CAD build for the part. Positions are in the model's coordinates, mm. A direction names the side the tool comes from. Round coordinates to 2 decimals unless told otherwise and drop trailing zeros. Write each loop counter-clockwise with the first axis right and the second up, starting at its lowest first coordinate (ties: lowest second). Pieces come first, ordered by that corner, then holes. Notation, with made-up numbers: (42, -35) - (84, -35) arc R12 ccw to (84, -27) - close; hole circle Ø1 at (80, 78.5). An arc over 180 degrees is marked (long way). Answer in a Markdown table with one row per item.
```python
from build123d import *

# Parameters (mm, degrees)
F0_R        = 10.025
F0_R_2      = 4.5
F1_DEPTH    = 1.5
F0_R_3      = 11.025
F1_FACE_R   = 10.025
F1_FACE_R_2 = 4.5
F2_DEPTH    = 2
F3_DEPTH    = 2
F4_DEPTH    = 1.5
F5_DEPTH    = 1.5
F6_DEPTH    = 2
F7_DEPTH    = 1.5


with BuildPart() as f1:
    # F0 (on Top) → F1 (new body)
    with BuildSketch(Plane.XY):
        Circle(F0_R)
        Circle(F0_R_2, mode=Mode.SUBTRACT)
    extrude(amount=F1_DEPTH)

    # F0 (on Top) + F1_face (on face) → F2 (join)
    with BuildSketch(Plane.XY):
        Circle(F0_R_3)
        Circle(F0_R, mode=Mode.SUBTRACT)
    with BuildSketch(Plane(origin=(0, 0, 0), x_dir=(1, 0, 0), z_dir=(0, 0, -1))):
        Circle(F1_FACE_R)
        Circle(F1_FACE_R_2, mode=Mode.SUBTRACT)
    extrude(amount=F2_DEPTH, dir=(0, 0, 1))

    # F0 (on Top) → F3 (join)
    with BuildSketch(Plane.XY):
        Circle(F0_R_3)
        Circle(F0_R, mode=Mode.SUBTRACT)
    extrude(amount=-F3_DEPTH)

    # F4 (add): a face of the model
    f4_faces = [f1.faces().sort_by_distance(p)[0] for p in [
        (-9.7414501807, 0, 0),
    ]]
    extrude(f4_faces, amount=F4_DEPTH)

    # F5 (add): a face of the model
    f5_faces = [f1.faces().sort_by_distance(p)[0] for p in [
        (-9.7414501807, 0, -1.5),
    ]]
    extrude(f5_faces, amount=F5_DEPTH)

    # F6 (add): a face of the model
    f6_faces = [f1.faces().sort_by_distance(p)[0] for p in [
        (-10.7131659095, 0, -2),
    ]]
    extrude(f6_faces, amount=F6_DEPTH)

    # F0 (on Top) → F7 (join)
    with BuildSketch(Plane.XY):
        Circle(F0_R)
        Circle(F0_R_2, mode=Mode.SUBTRACT)
    extrude(amount=-F7_DEPTH)


solid = f1.part
```
Q1. Drill centre lines: line 1 (Y direction, x = 0, z = -1.25) (3 decimals); line 2 (Z direction, x = 5.5, y = 4); line 3 (X direction, y = -1.5, z = 1.3). Where is each one in solid material? Low to high.
Computed:
| item | result |
|---|---|
| line 1 | y = -11.025 to -4.5, 4.5 to 11.025 |
| line 2 | z = -3 to 2 |
| line 3 | x = -10.92 to -4.24, 4.24 to 10.92 |
Q2. Saw through at A-A on y = 0. List the corners of the cut face in (x, z) (3 decimals), then the cut area to 4 significant figures.
Computed:
| item | result |
|---|---|
| outline | (-11.025, -4) - (-10.025, -4) - (-10.025, -3) - (-4.5, -3) - (-4.5, 2) - (-11.025, 2) - close; (4.5, -3) - (10.025, -3) - (10.025, -4) - (11.025, -4) - (11.025, 2) - (4.5, 2) - close |
| area | 67.25 mm2 |
Q3. Saw through at C-C on z = 0.7. List the corners of the cut face in (x, y) (3 decimals), then the cut area to 3 significant figures.
Computed:
| item | result |
|---|---|
| outline | circle Ø22.05 at (0, 0); hole circle Ø9 at (0, 0) |
| area | 318 mm2 |
Q4. Pull direction Y, two halves, no side cores. Call faces 1 (the cylindrical face through (-2.39, -10.763, -0.958)), 2 (the cylindrical face through (-0.59, 4.46, -0.46)), 3 (the flat face through (2, -10, -4)), 4 (the cylindrical face through (-7.955, -6.1, -3.493)): released by +Y, released by -Y, zero draft, split by the parting line, or undercut.
Computed:
| item | result |
|---|---|
| face 1 | split by the parting line |
| face 2 | undercut |
| face 3 | zero draft |
| face 4 | undercut |
Q5. Flat gauge pins, fed straight in: pin 1 (1.5 mm diameter, centred on y = 4.5, z = -0.5, fed in from -X); pin 2 (1.5 mm diameter, centred on x = 0.5, z = -1.5, fed in from -Y) (3 decimals); pin 3 (2 mm diameter, centred on y = -6, z = -2, fed in from -X); pin 4 (2 mm diameter, centred on y = -4.5, z = -1.5, fed in from -X). Where does each tip first touch, or does it go through?
Computed:
| item | result |
|---|---|
| pin 1 | stops at x = -10.37 |
| pin 2 | stops at y = -11.025 |
| pin 3 | stops at x = -9.83 |
| pin 4 | stops at x = -10.45 |
Q6. Saw through at D-D on x = -7. List the corners of the cut face in (y, z).
Computed:
| item | result |
|---|---|
| outline | (-8.52, -4) - (-7.18, -4) - (-7.18, -3) - (7.18, -3) - (7.18, -4) - (8.52, -4) - (8.52, 2) - (-8.52, 2) - close |
Q7. 3-axis set-ups, long thin cutter, end or side, ignore diameter. For faces 5 (the flat face through (5, 0, 2)), 6 (the flat face through (2.1, -4.3, -3)): which of +Z, -Z, +X, -X, +Y, -Y reach the whole face in a straight line?
Computed:
| item | result |
|---|---|
| face 5 | +Z, +X, -X, +Y, -Y |
| face 6 | -Z |
